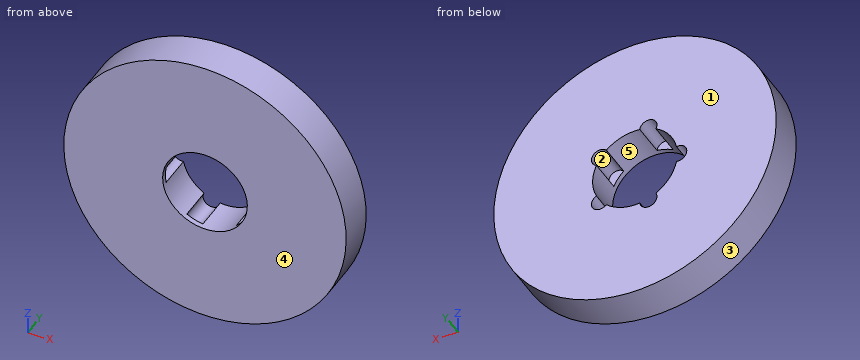
from build123d import *

# Parameters (mm, degrees)
SKETCH1_R           = 100
BOSS_EXTRUDE1_DEPTH = 27
SKETCH2_R           = 30
CUT_EXTRUDE1_DEPTH  = 144.975692393
SKETCH3_R           = 6.103815366
CUT_EXTRUDE2_DEPTH  = 23.355243
CIRPATTERN1_START   = 3.644756843
CIRPATTERN1_DEPTH   = 23.355243157


# Read off the part's stored shape, not the designer's step: CirPattern1
with BuildPart() as part:
    # Sketch1 → Boss-Extrude1 (new body)
    with BuildSketch(Plane(origin=(0, 0, 0), x_dir=(1, 0, 0), z_dir=(0, 1, 0))):
        with Locations(Location((0, 0, 0), (0, 0, 270))):
            Circle(SKETCH1_R)
    extrude(amount=BOSS_EXTRUDE1_DEPTH)

    # Sketch2 → Cut-Extrude1 (cut, through all)
    with BuildSketch(Plane(origin=(0, 0, 0), x_dir=(1, 0, 0), z_dir=(0, 1, 0))):
        with Locations(Location((0, 0, 0), (0, 0, 270))):
            Circle(SKETCH2_R)
    extrude(amount=CUT_EXTRUDE1_DEPTH, mode=Mode.SUBTRACT)

    # Sketch3 → Cut-Extrude2 (cut)
    with BuildSketch(Plane(origin=(0, 27, 0), x_dir=(1, 0, 0), z_dir=(0, 1, 0))):
        with Locations((-30.591261491, 0)):
            Circle(SKETCH3_R)
    extrude(amount=-CUT_EXTRUDE2_DEPTH, mode=Mode.SUBTRACT)

    # CirPattern1 outline → CirPattern1 (cut)
    with BuildSketch(Plane(origin=(0, 0, 0), x_dir=(1, 0, 0), z_dir=(0, 1, 0)).offset(CIRPATTERN1_START)):
        with BuildLine():
            ThreePointArc((-3.391271665, -29.807704985), (-9.270509831, -28.531695489), (-14.776932985, -26.108279368))
            ThreePointArc((-14.776932985, -26.108279368), (-11.339402358, -34.899091961), (-3.391271665, -29.807704985))
        make_face()
        with BuildLine():
            ThreePointArc((-3.391271665, 29.807704985), (-11.339402358, 34.899091961), (-14.776932985, 26.108279368))
            ThreePointArc((-14.776932985, 26.108279368), (-9.270509831, 28.531695489), (-3.391271665, 29.807704985))
        make_face()
        with BuildLine():
            ThreePointArc((27.300851485, -12.436378419), (24.270509831, -17.633557568), (20.264125805, -22.121600425))
            ThreePointArc((20.264125805, -22.121600425), (29.686940787, -21.568825008), (27.300851485, -12.436378419))
        make_face()
        with BuildLine():
            ThreePointArc((27.300851485, 12.436378419), (29.686940787, 21.568825008), (20.264125805, 22.121600425))
            ThreePointArc((20.264125805, 22.121600425), (24.270509831, 17.633557568), (27.300851485, 12.436378419))
        make_face()
    extrude(amount=CIRPATTERN1_DEPTH, mode=Mode.SUBTRACT)


solid = part.part
For this review, take the finished solid that the model builds, in its own axes (mm). Face numbers are marked on the shaded views. A direction names the side the tool comes from. Round coordinates to 2 decimals unless told otherwise and drop trailing zeros. Loops run counter-clockwise (first coordinate to the right, second up) from the corner with the lowest first, then second, coordinate; pieces in that order, holes last. Notation, with made-up numbers: (2, 51) - (6, 51) arc R32 ccw to (6, 79) - close; hole circle Ø4 at (26, -11). An arc over 180 degrees is marked (long way). Put each result on its own line as item: value. Start each with the question number.
1. For probe 1 along X at (y, z) = (25.25, 33.5); probe 2 along X at (y, z) = (21.25, -31); probe 3 along X at (y, z) = (6.5, 37.5), list the stretches that pass through material, from the lowest coordinate up. Write a range as [from, to].
2. Consider section A-A on z = 0. State the section outline as (x, y) points.
3. For the marked faces 1 and 2, list the 3-axis set-ups (+Z, -Z, +X, -X, +Y, -Y) from which the entire face can be reached by the end or side of a thin tool; tool diameter is ignored.
4. Consider section C-C on y = 12. State the section outline as (x, z) points.
5. Mouldability with a two-part tool opening along Z and no side actions: class the marked faces 3, 4 and 5 as +Z half, -Z half, draft (parallel to the pull), parting line (faces both ways), or undercut.
6. Consider section B-B on x = 0. State the section outline as (y, z) points.
7. Insertion check: P1, Ø8, axis at x = 63.5, y = 11.5, coming from the +Z side; P2, Ø10, axis at x = -9.45, z = -29.09, coming from the +Y side; P3, Ø4, axis at x = -6.5, y = 18.5, coming from the +Z side. Each pin has a flat end and moves straight along its axis. Give the tip position at first contact, or say it passes through.
8. Consider section D-D on z = 58. State the section outline as (x, y) points, plus the area to 3 significant figures.
Result sheet:
1. probe 1: [-94.22, -13.68], [-5.23, 94.22]
1. probe 2: [-95.07, -15.25], [-3.65, 95.07]
1. probe 3: [-92.7, 92.7]
2. outline: (-100, 0) - (-30, 0) - (-30, 3.64) - (-36.7, 3.64) - (-36.7, 27) - (-100, 27) - close; (30, 0) - (100, 0) - (100, 27) - (30, 27) - close
3. face 1: +Z, -Z, +X, -X, +Y
3. face 2: +Y
4. outline: circle Ø200 at (0, 0); hole (-29.4, -5.99) arc R30 ccw to (-14.78, -26.11) arc R6.1 ccw (long way) to (-3.39, -29.81) arc R30 ccw to (20.26, -22.12) arc R6.1 ccw (long way) to (27.3, -12.44) arc R30 ccw to (27.3, 12.44) arc R6.1 ccw (long way) to (20.26, 22.12) arc R30 ccw to (-3.39, 29.81) arc R6.1 ccw (long way) to (-14.78, 26.11) arc R30 ccw to (-29.4, 5.99) arc R6.1 ccw (long way) to start
5. face 3: parting line
5. face 4: draft
5. face 5: undercut
6. outline: (0, -100) - (27, -100) - (27, -30) - (0, -30) - close; (0, 30) - (27, 30) - (27, 100) - (0, 100) - close
7. P1: z = 80.37
7. P2: y = 3.64
7. P3: z = 99.9
8. outline: (-81.46, 0) - (81.46, 0) - (81.46, 27) - (-81.46, 27) - close
8. area: 4,400 mm^2
